Can you work these out from the model? Positions are in its coordinate system, mm. A direction names the side the tool comes from. Round coordinates to 2 decimals unless told otherwise and drop trailing zeros. Order: outer loops, then holes, each group sorted by start corner. A loop starts at its lowest first (then second) coordinate and runs counter-clockwise, first axis right, second up. Notation, with made-up numbers: (-3, -9) -> (48, -9) arc R12 ccw to (48, 7) -> close; hole circle Ø1 at (-4.5, -8.5). An arc over 180 degrees is marked (long way). One line per item, written item: value.
```python
from build123d import *

# Parameters (mm, degrees)
SKETCH2_R            = 3
BOSS_EXTRUDE1_DEPTH  = 81.5
SKETCH4_R            = 4
BOSS_EXTRUDE2_DEPTH  = 5
CUT_EXTRUDE1_DEPTH   = 4
FILLET1_R            = 0.1
FILLET1_OF_MIRROR1_R = 0.1


with BuildPart() as part:
    # Sketch2 → Boss-Extrude1 (new body, symmetric)
    with BuildSketch(Plane(origin=(0, 0, 0), x_dir=(1, 0, 0), z_dir=(0, 1, 0))):
        Circle(SKETCH2_R)
    extrude(amount=BOSS_EXTRUDE1_DEPTH, both=True)

    # Sketch4 → Boss-Extrude2 (add)
    with BuildSketch(Plane(origin=(0, 81.5, 0), x_dir=(1, 0, 0), z_dir=(0, 1, 0))):
        Circle(SKETCH4_R)
    boss_extrude2 = extrude(amount=BOSS_EXTRUDE2_DEPTH)

    # Sketch5 → Cut-Extrude1 (cut)
    with BuildSketch(Plane(origin=(0, 86.5, 0), x_dir=(1, 0, 0), z_dir=(0, 1, 0))):
        Polygon((1.443375673, -2.5), (2.886751346, 0), (1.443375673, 2.5), (-1.443375673, 2.5), (-2.886751346, 0), (-1.443375673, -2.5), align=None)
    cut_extrude1 = extrude(amount=-CUT_EXTRUDE1_DEPTH, mode=Mode.SUBTRACT)

    # Fillet1
    fillet1_edges = [part.edges().sort_by_distance(p)[0] for p in [
        (0, 82.5, 2.5),
        (-2.165063509, 82.5, 1.25),
        (-2.165063509, 82.5, -1.25),
        (0, 82.5, -2.5),
        (2.165063509, 82.5, -1.25),
        (2.165063509, 82.5, 1.25),
        (0, 86.5, 2.5),
        (2.165063509, 86.5, 1.25),
        (2.165063509, 86.5, -1.25),
        (0, 86.5, -2.5),
        (-2.165063509, 86.5, -1.25),
        (-2.165063509, 86.5, 1.25),
        (-4, 86.5, 0),
    ]]
    fillet(fillet1_edges, radius=FILLET1_R)

    # Mirror1: Boss-Extrude2, Cut-Extrude1 across plane
    add(boss_extrude2.mirror(Plane.ZX))
    add(cut_extrude1.mirror(Plane.ZX), mode=Mode.SUBTRACT)

    # Fillet1 of Mirror1
    fillet1_of_mirror1_edges = [part.edges().sort_by_distance(p)[0] for p in [
        (0, -82.5, 2.5),
        (-2.165063509, -82.5, 1.25),
        (-2.165063509, -82.5, -1.25),
        (0, -82.5, -2.5),
        (2.165063509, -82.5, -1.25),
        (2.165063509, -82.5, 1.25),
        (0, -86.5, 2.5),
        (2.165063509, -86.5, 1.25),
        (2.165063509, -86.5, -1.25),
        (0, -86.5, -2.5),
        (-2.165063509, -86.5, -1.25),
        (-2.165063509, -86.5, 1.25),
        (-4, -86.5, 0),
    ]]
    fillet(fillet1_of_mirror1_edges, radius=FILLET1_OF_MIRROR1_R)


solid = part.part
```
Q1. We'd pull the mould along Y, two halves only. Please class faces 4 (the face through (0, -82.5, 0)), 5 (the face through (-0.867, 83.916, 3.905)), 6 (the face through (1, -81.5, -3)): released by +Y, released by -Y, zero draft, split by the parting line, or undercut.
Answers below:
face 4: released by -Y
face 5: zero draft
face 6: undercut
Q2. Please list where these lines run through material, in increasing order: line 1 along Y through (x, z) = (3.25, -0.5); line 2 along Z through (x, y) = (-0.75, -45.5); line 3 along Y through (x, z) = (-0.75, -2.25).
Answers below:
line 1: -86.5 to -81.5, 81.5 to 86.5
line 2: -2.9 to 2.9
line 3: -82.5 to 82.5
Q3. Will these pins go through, and if not, where does the flat tip stop? pin 1 Ø4 at (x, y) = (-1, -8) entering from +Z; pin 2 Ø1 at (y, z) = (24, -2) entering from +X; pin 3 Ø1.5 at (y, z) = (39, 0) entering from -X.
Answers below:
pin 1: z = 3
pin 2: x = 2.6
pin 3: x = -3
Q4. On a 3-axis mill with a long thin cutter (end or side, diameter ignored), from which of +Z, -Z, +X, -X, +Y, -Y can I reach the whole of each face in a straight line? I mean faces 1 (the face through (0, -85, 2.5)), 2 (the face through (1, 81.5, -3)), 3 (the face through (0, 85, -2.5)). Say none if no direction works.
Answers below:
face 1: -Y
face 2: none
face 3: +Y
Q5. I want a section at B-B on y = -69. List the corners of the cut face in (x, z) for me, plus the area to 3 significant figures.
Answers below:
outline: circle Ø6 at (0, 0)
area: 28.3 mm^2
